from build123d import *

# Parameters (mm, degrees)
BOSS_EXTRUDE1_DEPTH = 24
SKETCH2_R           = 4
SKETCH2_R_2         = 1.5
CUT_EXTRUDE1_DEPTH  = 4
SKETCH3_R           = 4
SKETCH3_R_2         = 1.5
CUT_EXTRUDE2_DEPTH  = 4
FILLET1_R           = 4
SKETCH6_R           = 4
SKETCH6_R_2         = 1.5
CUT_EXTRUDE3_DEPTH  = 4


with BuildPart() as part:
    # Sketch1 → Boss-Extrude1 (new body)
    with BuildSketch(Plane.XY):
        Polygon((-35.947712149, -38.738038278), (-35.947712149, 36.261961722), (20.052287851, 36.261961722), (20.052287851, -38.738038278), (24.052287851, -38.738038278), (24.052287851, 40.261961722), (-39.947712149, 40.261961722), (-39.947712149, -38.738038278), align=None)
    extrude(amount=BOSS_EXTRUDE1_DEPTH)

    # Sketch2 → Cut-Extrude1 (cut)
    with BuildSketch(Plane(origin=(24.052287851, 0, 0), x_dir=(0, 0, -1), z_dir=(1, 0, 0))):
        with Locations((-12, -26.738038278)):
            Circle(SKETCH2_R)
        with Locations((-4, -26.738038278)):
            Circle(SKETCH2_R_2)
        with Locations((-12, -34.738038278)):
            Circle(SKETCH2_R_2)
        with Locations((-20, -26.738038278)):
            Circle(SKETCH2_R_2)
        with Locations((-12, -18.738038278)):
            Circle(SKETCH2_R_2)
    extrude(amount=-CUT_EXTRUDE1_DEPTH, mode=Mode.SUBTRACT)

    # Sketch3 → Cut-Extrude2 (cut)
    with BuildSketch(Plane.ZY.offset(39.947712149)):
        with Locations((12, -26.738038278)):
            Circle(SKETCH3_R)
        with Locations((20, -26.738038278)):
            Circle(SKETCH3_R_2)
        with Locations((12, -34.738038278)):
            Circle(SKETCH3_R_2)
        with Locations((4, -26.738038278)):
            Circle(SKETCH3_R_2)
        with Locations((12, -18.738038278)):
            Circle(SKETCH3_R_2)
    extrude(amount=-CUT_EXTRUDE2_DEPTH, mode=Mode.SUBTRACT)

    # Fillet1
    fillet1_edges = [part.edges().sort_by_distance(p)[0] for p in [
        (22.052287851, -38.738038278, 0),
        (20.052287851, 36.261961722, 12),
        (-35.947712149, 36.261961722, 12),
        (-39.947712149, 40.261961722, 12),
        (24.052287851, 40.261961722, 12),
        (-37.947712149, -38.738038278, 24),
        (22.052287851, -38.738038278, 24),
        (-37.947712149, -38.738038278, 0),
    ]]
    fillet(fillet1_edges, radius=FILLET1_R)

    # Sketch6 → Cut-Extrude3 (cut)
    with BuildSketch(Plane(origin=(0, 40.261961722, 0), x_dir=(1, 0, 0), z_dir=(0, 1, 0))):
        with Locations((-7.947712149, -12)):
            Circle(SKETCH6_R)
        with Locations((0.052287851, -12)):
            Circle(SKETCH6_R_2)
        with Locations((-7.947712149, -20)):
            Circle(SKETCH6_R_2)
        with Locations((-15.947712149, -12)):
            Circle(SKETCH6_R_2)
        with Locations((-7.947712149, -4)):
            Circle(SKETCH6_R_2)
    extrude(amount=-CUT_EXTRUDE3_DEPTH, mode=Mode.SUBTRACT)


solid = part.part
Can you work these out from the model? Positions are in its coordinate system, mm. A direction names the side the tool comes from. Round coordinates to 2 decimals unless told otherwise and drop trailing zeros. Write each loop counter-clockwise with the first axis right and the second up, starting at its lowest first coordinate (ties: lowest second). Pieces come first, ordered by that corner, then holes. Notation, with made-up numbers: (-36, -5.75) -> (5, -5.75) arc R30 cw to (5, 33.25) -> close; hole circle Ø5 at (58, -22.5). An arc over 180 degrees is marked (long way). One line per question, with ' | ' between items. Start each with the question number.
1) Suppose I cut it at B-B on y = -24. Write out the boundary of the cut face in (x, z), then the cut area to 3 significant figures.
2) I'm going to push a flat-ended pin straight in: P1, Ø5, axis at x = -15.95, z = 12, coming from the -Y side. Where does the tip first touch, or does it pass through?
3) Suppose I cut it at D-D on x = -20.5. Write out the boundary of the cut face in (y, z), then the cut area to 3 significant figures.
4) On a 3-axis mill with a long thin cutter (end or side, diameter ignored), from which of +Z, -Z, +X, -X, +Y, -Y can I reach the whole of each face in a straight line? I mean faces 4 (the flat face through (-35.948, -4, 12)), 5 (the cylindrical face through (-37.98, -20.2, 11.67)). Say none if no direction works.
5) I need wall thicknesses on line 1 (X direction, y = -34, z = 8.25); line 2 (X direction, y = 33.5, z = 3.5); line 3 (Y direction, x = 22.6, z = 12). Which ranges of each line are inside material? Lowest first, please. Write a range as [from, to].
6) Suppose I cut it at C-C on z = 12. Count the separate pieces of the cut face and the enclosed holes in it, then the cut area to 3 significant figures.
7) If we mould it in two halves opening along X, with no side actions, what happens to faces 1 (the cylindrical face through (22.08, -20.2, 12.33)), 2 (the flat face through (-3, 36.262, 12)), 3 (the cylindrical face through (-38.807, 39.059, 12.168))? For each: released by +X, released by -X, zero draft, split by the parting line, or undercut.
8) Suppose I cut it at A-A on y = -13.5. Write out the boundary of the cut face in (x, z), then the cut area to 3 significant figures.
Return value:
1) outline: (-39.95, 0) -> (-35.95, 0) -> (-35.95, 9.08) -> (-39.95, 9.08) -> close; (-39.95, 14.92) -> (-35.95, 14.92) -> (-35.95, 24) -> (-39.95, 24) -> close; (20.05, 0) -> (24.05, 0) -> (24.05, 9.08) -> (20.05, 9.08) -> close; (20.05, 14.92) -> (24.05, 14.92) -> (24.05, 24) -> (20.05, 24) -> close | area: 145 mm2
2) P1: stops at y = 36.26
3) outline: (36.26, 0) -> (40.26, 0) -> (40.26, 24) -> (36.26, 24) -> close | area: 96.0 mm2
4) face 4: +Z, -Z, -Y | face 5: +X, -X
5) line 1: x = [-39.95, -35.95], [20.05, 24.05] | line 2: x = [-39.95, -35.75], [19.86, 24.05] | line 3: y = [-38.74, -36.24], [-33.24, -30.74], [-22.74, -20.24], [-17.24, 39.35]
6) separate pieces: 10 | enclosed holes: 0 | area: 688 mm2
7) face 1: zero draft | face 2: undercut | face 3: released by -X
8) outline: (-39.95, 0) -> (-35.95, 0) -> (-35.95, 24) -> (-39.95, 24) -> close; (20.05, 0) -> (24.05, 0) -> (24.05, 24) -> (20.05, 24) -> close | area: 192 mm2
